```python
from build123d import *
from build123d.topology import SkipClean

# Parameters (mm, degrees)
RESSALTO_EXTRUS_O1_DEPTH = 1.4
ESBO_O2_R                = 3.45
RESSALTO_EXTRUS_O2_DEPTH = 2
ESBO_O3_R                = 2.25
CORTE_EXTRUS_O1_DEPTH    = 2
CORTE_EXTRUS_O2_START    = -0.5
ESBO_O4_R                = 2.25
CORTE_EXTRUS_O2_DEPTH    = 0.5
ESBO_O5_R                = 1.25
CORTE_EXTRUS_O3_DEPTH    = 17.62265021
ESBO_O6_R                = 0.5
CORTE_EXTRUS_O4_DEPTH    = 17.717131931


with BuildPart() as part:
    # Esboço1 → Ressalto-extrusão1 (new body)
    with BuildSketch(Plane(origin=(0, 0, 0), x_dir=(1, 0, 0), z_dir=(0, 1, 0))):
        with BuildLine():
            Line((-14.101708317, 1.99741218), (-2.267708094, 2.6))
            ThreePointArc((-2.267708094, 2.6), (0, 3.45), (2.267708094, 2.6))
            Line((2.267708094, 2.6), (14.101708317, 1.99741218))
            ThreePointArc((14.101708317, 1.99741218), (16, 0), (14.101708317, -1.99741218))
            Line((14.101708317, -1.99741218), (2.267708094, -2.6))
            ThreePointArc((2.267708094, -2.6), (0, -3.45), (-2.267708094, -2.6))
            Line((-2.267708094, -2.6), (-14.101708317, -1.99741218))
            ThreePointArc((-14.101708317, -1.99741218), (-16, 0), (-14.101708317, 1.99741218))
        make_face()
    extrude(amount=RESSALTO_EXTRUS_O1_DEPTH)

    # Esboço2 → Ressalto-extrusão2 (add)
    with SkipClean():  # the faces are left unmerged after this step: merging them gives an invalid solid
        with BuildSketch(Plane(origin=(0, 1.4, 0), x_dir=(1, 0, 0), z_dir=(0, 1, 0))):
            with Locations(Location((0, 0, 0), (0, 0, 48.905212005))):
                Circle(ESBO_O2_R)
        extrude(amount=RESSALTO_EXTRUS_O2_DEPTH)

    # Esboço3 → Corte-extrusão1 (cut)
    with SkipClean():  # the faces are left unmerged after this step: merging them gives an invalid solid
        with BuildSketch(Plane(origin=(0, 3.4, 0), x_dir=(1, 0, 0), z_dir=(0, 1, 0))):
            with Locations(Location((0, 0, 0), (0, 0, 270))):
                Circle(ESBO_O3_R)
        extrude(amount=-CORTE_EXTRUS_O1_DEPTH, mode=Mode.SUBTRACT)

    # Esboço4 → Corte-extrusão2 (cut)
    with SkipClean():  # the faces are left unmerged after this step: merging them gives an invalid solid
        with BuildSketch(Plane.XZ.offset(CORTE_EXTRUS_O2_START)):
            with Locations(Location((0, 0, 0), (0, 0, 90))):
                Circle(ESBO_O4_R)
        extrude(amount=CORTE_EXTRUS_O2_DEPTH, mode=Mode.SUBTRACT)

    # Esboço5 → Corte-extrusão3 (cut, through all)
    with SkipClean():  # the faces are left unmerged after this step: merging them gives an invalid solid
        with BuildSketch(Plane.XZ.offset(-0.5)):
            with Locations(Location((0, 0, 0), (0, 0, 270))):
                Circle(ESBO_O5_R)
        extrude(amount=-CORTE_EXTRUS_O3_DEPTH, mode=Mode.SUBTRACT)

    # Esboço6 → Corte-extrusão4 (cut, through all)
    with SkipClean():  # the faces are left unmerged after this step: merging them gives an invalid solid
        with BuildSketch(Plane.XZ):
            with Locations(Location((-4, 0, 0), (0, 0, 270))):
                Circle(ESBO_O6_R)
            with Locations(Location((-6, 0, 0), (0, 0, 270))):
                Circle(ESBO_O6_R)
            with Locations(Location((-8, 0, 0), (0, 0, 270))):
                Circle(ESBO_O6_R)
            with Locations(Location((-10, 0, 0), (0, 0, 270))):
                Circle(ESBO_O6_R)
            with Locations(Location((-12, 0, 0), (0, 0, 270))):
                Circle(ESBO_O6_R)
            with Locations(Location((-14, 0, 0), (0, 0, 270))):
                Circle(ESBO_O6_R)
        corte_extrus_o4 = extrude(amount=-CORTE_EXTRUS_O4_DEPTH, mode=Mode.SUBTRACT)

    # Espelhar1: Corte-extrusão4 across plane
    with SkipClean():  # the faces are left unmerged after this step: merging them gives an invalid solid
        add(corte_extrus_o4.mirror(Plane(origin=(0, 0, 0), x_dir=(0, 0, 1), z_dir=(1, 0, 0))), mode=Mode.SUBTRACT)


solid = part.part
```
Source: CAD feature listing. Evaluate the final solid. Frame: model axes, mm. A direction names the side the tool comes from. Round coordinates to 2 decimals unless told otherwise and drop trailing zeros. Loops run counter-clockwise (first coordinate to the right, second up) from the corner with the lowest first, then second, coordinate; pieces in that order, holes last. Notation, with made-up numbers: M 43,28 L 68,28 A11 ccw 68,36 Z; hole C 6,38.5 d7. An arc over 180 degrees is marked long. Use a Markdown table: item, result. Add a question column.
1. Line query: line 1 (Z direction, x = 14, y = 0.35); line 2 (Y direction, x = 6.5, z = 2.25); line 3 (X direction, y = 2.35, z = 1). Output: solid intervals per line, ascending.
2. Reachability of faces 1 (the flat face through (8.102, 0.69, -2.303)), 2 (the flat face through (-1, 1.4, 1)), 3 (the cylindrical face through (-0.676, 0.254, 2.146)) from +Z, -Z, +X, -X, +Y, -Y: full face, straight path, thin tool, end or side. Return the list, or none.
3. Section query D-D on x = 6. Return the cut outline in (y, z).
4. Section query C-C on x = 10. Return the cut outline in (y, z), then the cut area to 3 significant figures.
5. Section query A-A on x = 0. Return the cut outline in (y, z), then the cut area to 3 significant figures.
6. Mould query, pull axis Z, two halves, no side actions, for faces 4 (the cylindrical face through (16, 1, 0)), 5 (the cylindrical face through (-8.488, 0.69, 0.108)), 6 (the flat face through (-8.102, 0.69, 2.303)). Classes: pulls with the +Z half, pulls with the -Z half, needs draft (parallel to the pull), parting line crosses it, or undercut.
7. Contact query for flat-ended pins moving along their axis: P1, Ø2, axis at x = 7, y = 0.5, coming from the +Z side; P2, Ø3, axis at x = 0, z = 0, coming from the -Y side; P3, Ø1.5, axis at x = 4.5, y = 2, coming from the -Z side. Output: stop coordinate, or through.
8. Section query B-B on y = 2.15. Return the cut outline in (x, z), then the cut area to 3 significant figures.
Reported:
| question | item | result |
|---|---|---|
| 1 | line 1 | z = -2 to -0.5, 0.5 to 2 |
| 1 | line 2 | y = 0 to 1.4 |
| 1 | line 3 | x = -3.3 to -2.02, 2.02 to 3.3 |
| 2 | face 1 | -Z, +X, +Y, -Y |
| 2 | face 2 | +Y |
| 2 | face 3 | -Y |
| 3 | outline | M 0,-2.41 L 1.4,-2.41 L 1.4,-0.5 L 0,-0.5 Z; M 0,0.5 L 1.4,0.5 L 1.4,2.41 L 0,2.41 Z |
| 4 | outline | M 0,-2.21 L 1.4,-2.21 L 1.4,-0.5 L 0,-0.5 Z; M 0,0.5 L 1.4,0.5 L 1.4,2.21 L 0,2.21 Z |
| 4 | area | 4.78 mm² |
| 5 | outline | M 0,-3.45 L 3.4,-3.45 L 3.4,-2.25 L 1.4,-2.25 L 1.4,-1.25 L 0.5,-1.25 L 0.5,-2.25 L 0,-2.25 Z; M 0,2.25 L 0.5,2.25 L 0.5,1.25 L 1.4,1.25 L 1.4,2.25 L 3.4,2.25 L 3.4,3.45 L 0,3.45 Z |
| 5 | area | 9.96 mm² |
| 6 | face 4 | parting line crosses it |
| 6 | face 5 | undercut |
| 6 | face 6 | pulls with the +Z half |
| 7 | P1 | stops at z = 2.41 |
| 7 | P2 | stops at y = 0.5 |
| 7 | P3 | stops at z = -2.51 |
| 8 | outline | C 0,0 d6.9; hole C 0,0 d4.5 |
| 8 | area | 21.5 mm² |
